Read the model definition and answer for the solid it produces. Units are mm, in the model's axes. A direction names the side the tool comes from. Coordinates: 2 decimals unless noted, no trailing zeros. Write each loop counter-clockwise with the first axis right and the second up, starting at its lowest first coordinate (ties: lowest second). Pieces come first, ordered by that corner, then holes.
from build123d import *

# Parameters (mm, degrees)
CYLINDER022_R             = 2.3
CYLINDER022_DEPTH         = 12
CHAMFER002_SIZE           = 0.35
CYLINDER021_R             = 2.5
CYLINDER021_DEPTH         = 3
CYLINDER020_R             = 4
CYLINDER020_DEPTH         = 6
CHAMFER001_SIZE2          = 1.5
CHAMFER001_SIZE           = 5.98
CYLINDER019_R             = 1.5
CYLINDER019_DEPTH         = 10
FUSION005_ROLL_ANGLE      = 90
FUSION005_PLACEMENT_ANGLE = 180


with BuildPart() as chamfer002:
    # Cylinder022 → Cylinder022 (new body)
    with BuildSketch(Plane.XY.offset(39)):
        Circle(CYLINDER022_R)
    extrude(amount=CYLINDER022_DEPTH)

    # Chamfer002
    chamfer002_edges = [chamfer002.edges().sort_by_distance(p)[0] for p in [
        (-2.3, 0, 51),
    ]]
    chamfer(chamfer002_edges, length=CHAMFER002_SIZE)


with BuildPart() as cylinder021:
    # Cylinder021 → Cylinder021 (new body)
    with BuildSketch(Plane.XY.offset(36)):
        Circle(CYLINDER021_R)
    extrude(amount=CYLINDER021_DEPTH)


with BuildPart() as fusion003:
    # Cylinder020 → Cylinder020 (new body)
    with BuildSketch(Plane.XY):
        Circle(CYLINDER020_R)
    extrude(amount=CYLINDER020_DEPTH)

    # Chamfer001
    chamfer001_edges = [fusion003.edges().sort_by_distance(p)[0] for p in [
        (-4, 0, 6),
    ]]
    chamfer001_side = fusion003.faces().sort_by_distance((-4, 0, 3))[0]
    chamfer(chamfer001_edges, length=CHAMFER001_SIZE, length2=CHAMFER001_SIZE2, reference=chamfer001_side)


with BuildPart() as fusion003_1:
    # Chamfer001 placement: moved
    add(fusion003.part.moved(Location((0, 0, 30))))

    # Fusion003: union Cylinder021
    add(cylinder021.part)


with BuildPart() as rotor_shaft:
    # Cylinder019 → Cylinder019 (new body)
    with BuildSketch(Plane.XY.offset(28)):
        Circle(CYLINDER019_R)
    extrude(amount=CYLINDER019_DEPTH)

    # Fusion004: union Fusion003
    add(fusion003_1.part)

    # Fusion005: union Chamfer002
    add(chamfer002.part)


with BuildPart() as rotor_shaft_1:
    # Fusion005 roll: moved
    add(rotor_shaft.part.rotate(Axis((0, 0, 0), (1, 0, 0)), FUSION005_ROLL_ANGLE))


with BuildPart() as rotor_shaft_2:
    # Fusion005 placement: moved
    add(rotor_shaft_1.part.moved(Location((0, 20, 0))).rotate(Axis((0, 20, 0), (0, 0, 1)), FUSION005_PLACEMENT_ANGLE))


solid = rotor_shaft_2.part
Item 1: Given pin 1 (3 mm diameter, centred on y = 61.5, z = 0, fed in from +X); pin 2 (2 mm diameter, centred on x = 0, y = 61.5, fed in from -Z); pin 3 (2 mm diameter, centred on x = -2.5, y = 56.5, fed in from +Z), each flat-ended and moving along its own axis, determine where each tip first touches the part or whether it passes through.
Item 2: The part is cut by section D-D (y = 52.5). Give the vertices of the cut face in (x, z).
Item 3: The part is cut by section C-C (y = 63). Give the vertices of the cut face in (x, z).
Item 4: For faces 1 (the flat face through (-2, 50, 0)), 2 (the cylindrical face through (-2.385, 57.479, 0.751)), 3 (the flat face through (0, 71, 0)), determine the directions among +Z, -Z, +X, -X, +Y, -Y from which every point of the face is accessible in a straight line to the end or side of a thin tool.
Item 5: Find the intervals of material crossed by probe 1 along Z at (x, y) = (0.75, 68); probe 2 along X at (y, z) = (61.5, 0.25); probe 3 along X at (y, z) = (55.5, 0.25), in increasing order.
Answer:
1. pin 1: stops at x = 2.3
1. pin 2: stops at z = -2.3
1. pin 3: stops at z = 2
2. outline: circle Ø6.76 at (0, 0)
3. outline: circle Ø4.6 at (0, 0)
4. face 1: -Y
4. face 2: +Y
4. face 3: +Z, -Z, +X, -X, +Y
5. probe 1: z = -2.17 to 2.17
5. probe 2: x = -2.29 to 2.29
5. probe 3: x = -2.61 to 2.61
